```python
from build123d import *

# Parameters (mm, degrees)
F1_DEPTH = 1185


with BuildPart() as f1:
    # F0 (on Front) → F1 (new body, symmetric)
    with BuildSketch(Plane.XZ):
        with BuildLine():
            Line((0, 100), (0, 0))
            Line((0, 0), (7.5, 0))
            Line((7.5, 0), (7.5, 75.160644))
            ThreePointArc((7.5, 75.160644), (10.652672, 83.267727), (18.454131, 87.114981))
            Line((18.454131, 87.114981), (40, 89))
            Line((40, 89), (40, 100))
            Line((40, 100), (0, 100))
        make_face()
        with BuildLine():
            Line((80, 100), (40, 100))
            Line((40, 100), (40, 89))
            Line((40, 89), (74.522934, 92.020365))
            ThreePointArc((74.522934, 92.020365), (78.423664, 93.943992), (80, 97.997534))
            Line((80, 97.997534), (80, 100))
        make_face()
        with BuildLine():
            Line((7.5, 0), (0, 0))
            Line((0, 0), (0, -100))
            Line((0, -100), (40, -100))
            Line((40, -100), (40, -89))
            Line((40, -89), (18.454131, -87.114981))
            ThreePointArc((18.454131, -87.114981), (10.652672, -83.267727), (7.5, -75.160644))
            Line((7.5, -75.160644), (7.5, 0))
        make_face()
        with BuildLine():
            Line((40, -89), (40, -100))
            Line((40, -100), (80, -100))
            Line((80, -100), (80, -97.997534))
            ThreePointArc((80, -97.997534), (78.423664, -93.943992), (74.522934, -92.020365))
            Line((74.522934, -92.020365), (40, -89))
        make_face()
    extrude(amount=F1_DEPTH, both=True)


solid = f1.part
```
For this review, take the finished solid that the model builds, in its own axes (mm). Round coordinates to 2 decimals unless told otherwise and drop trailing zeros. Write each loop counter-clockwise with the first axis right and the second up, starting at its lowest first coordinate (ties: lowest second). Pieces come first, ordered by that corner, then holes.
1) Mouldability with a two-part tool opening along X and no side actions: class faces 1 (the face through (7.5, -17, -1)), 2 (the face through (41, -17, 100)), 3 (the face through (0, -17, 1)) as +X half, -X half, draft (parallel to the pull), parting line (faces both ways), or undercut.
Answer below:
face 1: +X half
face 2: draft
face 3: -X half
2) For line 1 along Z through (x, y) = (17, -759); line 2 along Z through (x, y) = (37, -1015.5); line 3 along X through (y, z) = (-287, 56), list the stretches that pass through material, from the lowest coordinate up.
Answer below:
line 1: z = -100 to -86.9, 86.9 to 100
line 2: z = -100 to -88.74, 88.74 to 100
line 3: x = 0 to 7.5
3) Take a section at B-B on y = -145. Give the boundary of the cut face in (x, z).
Answer below:
outline: (0, -100) - (80, -100) - (80, -98) arc R6 ccw to (74.52, -92.02) - (18.45, -87.11) arc R12 cw to (7.5, -75.16) - (7.5, 75.16) arc R12 cw to (18.45, 87.11) - (74.52, 92.02) arc R6 ccw to (80, 98) - (80, 100) - (0, 100) - close
4) Take a section at C-C on z = 6.5. Give the boundary of the cut face in (x, y).
Answer below:
outline: (0, -1185) - (7.5, -1185) - (7.5, 1185) - (0, 1185) - close
5) Insertion check: pin 1 Ø12 at (y, z) = (-711.5, -3.5) entering from +X. The pin has a flat end and moves straight along its axis. Give the tip position at first contact, or say it passes through.
Answer below:
pin 1: stops at x = 7.5
6) Take a section at A-A on x = 59. Give the boundary of the cut face in (y, z).
Answer below:
outline: (-1185, -100) - (1185, -100) - (1185, -90.66) - (-1185, -90.66) - close; (-1185, 90.66) - (1185, 90.66) - (1185, 100) - (-1185, 100) - close
